Build history of the part. All positions in model axes, mm. A direction names the side the tool comes from. Round coordinates to 2 decimals unless told otherwise and drop trailing zeros. Write each loop counter-clockwise with the first axis right and the second up, starting at its lowest first coordinate (ties: lowest second). Pieces come first, ordered by that corner, then holes. Notation, with made-up numbers: M 0,52 L 5,52 A24 cw 5,66 Z; hole C 74.5,75.5 d5. An arc over 180 degrees is marked long. Write item = value, one per line. Start each with the question number.
Q1. Band-saw the part on D-D on x = 62. Write the cut outline in (y, z).
Q2. Pull direction Y, two halves, no side cores. Call faces 1 (the flat face through (48, 10, 110)), 2 (the cylindrical face through (76.48, 12.87, 133.07)), 3 (the flat face through (0, 86, 8)): released by +Y, released by -Y, zero draft, split by the parting line, or undercut.
Q3. Band-saw the part on C-C on y = 79. Write the cut outline in (x, z), plus the area to 3 significant figures.
Q4. Band-saw the part on A-A on x = 21. Write the cut outline in (y, z), plus the area to 3 significant figures.
Q5. Probe L1, parallel to Y at x = 3.2, z = 30; L2, parallel to Y at x = 1.2, z = 5. List the from-to ranges inside material, lowest first.
Q6. Band-saw the part on B-B on z = 73.5. Write the cut outline in (x, y), plus the area to 3 significant figures.
Q7. Drop flat-ended pins along their axis: P1, Ø2.5, axis at x = 76, z = 34, coming from the +Y side; P2, Ø0.9, axis at x = 76.5, z = 99.5, coming from the -Y side; P3, Ø2.5, axis at y = 145.5, z = 120.5, coming from the -X side; P4, Ø0.9, axis at y = 12, z = 106.5, coming from the -X side. Give the stop position or say it passes through.
Q8. Tool access for faces 4 (the flat face through (50, 5, 110)), 5 (the cylindrical face through (76.48, 17.32, 11.63)), 6 (the flat face through (48, 17, 12)): list every direction of +Z, -Z, +X, -X, +Y, -Y with a clear straight run to the whole face (end or side of a thin tool).
Autodesk Inventor part; units mm, degrees
ref_plane "YZ Plane" through (0, 0, 0) normal (1, 0, 0) x (0, 1, 0)
ref_plane "XZ Plane" through (0, 0, 0) normal (0, 1, 0) x (-1, 0, 0)
ref_plane "XY Plane" through (0, 0, 0) normal (0, 0, 1) x (1, 0, 0)
sketch "Sketch1" plane through (0, 0, 0) normal (0, 0, 1) x (1, 0, 0)
  line L0 (0, 0) -> (75, 0)
  line L1 (75, 0) -> (75, 150)
  line L2 (75, 150) -> (0, 150)
  line L3 (0, 150) -> (0, 0)
  dimension "d0" = 75
  dimension "d1" = 150
extrude "Extrusion1" add sketch "Sketch1" along normal blind 10
sketch "Sketch2" plane through (0, 0, 10) normal (0, 0, 1) x (1, 0, 0)
  line L0 (48, 85) -> (53, 85)
  line L1 (53, 85) -> (53, 19)
  line L2 (53, 19) -> (48, 19)
  line L3 (48, 19) -> (48, 14)
  line L4 (48, 14) -> (58, 14)
  line L5 (58, 14) -> (58, 90)
  line L6 (58, 90) -> (48, 90)
  line L7 (75, 150) -> (0, 150)
  line L8 (0, 150) -> (0, 0)
  line L9 (48, 85) -> (48, 90)
  dimension "d4" = 10
  dimension "d5" = 76
  dimension "d6" = 66
  dimension "d8" = 60
  dimension "d9" = 5
  dimension "d10" = 10
  dimension "d11" = 53
  dimension "d12" = 5
  dimension "d13" = 5
extrude "Extrusion2" add sketch "Sketch2" along normal blind 5
sketch "Sketch3" plane through (53, 19, 10) normal (-1, 0, 0) x (0, 0, 1)
  line L0 (5, 66) -> (5, 0)
  line L1 (5, 66) -> (3, 66)
  line L2 (3, 66) -> (3, 56)
  line L3 (3, 56) -> (5, 56)
  line L4 (5, 56) -> (5, 66)
  line L5 (5, 0) -> (5, -5)
  line L6 (5, 0) -> (3, 0)
  line L7 (3, 0) -> (3, 10)
  line L8 (3, 10) -> (5, 10)
  line L9 (5, 10) -> (5, 0)
  point P0 (-10, -19)
  point P1 (5, 10)
  point P2 (5, 56)
  dimension "d16" = 2
  dimension "d17" = 10
  dimension "d18" = 10
  dimension "d19" = 2
extrude "Extrusion3" add sketch "Sketch3" along normal blind 3
sketch "Sketch4" plane through (0, 0, 10) normal (0, 0, 1) x (1, 0, 0)
  line L0 (0, 150) -> (0, 0)
  line L1 (0, 10) -> (65, 10)
  line L2 (65, 10) -> (65, 140)
  line L3 (65, 140) -> (0, 140)
  line L4 (75, 150) -> (0, 150)
  line L5 (75, 0) -> (75, 150)
  line L6 (0, 0) -> (75, 0)
  point P0 (0, 140)
  dimension "d22" = 10
  dimension "d24" = 10
  dimension "d25" = 10
extrude "Extrusion4" add sketch "Sketch4" along normal blind 140 contours L4 L5 L6 L0 L1 L2 L3
sketch "Sketch5" plane through (0, 10, 10) normal (0, 1, 0) x (1, 0, 0)
  line L0 (0, 10) -> (0, -140)
  line L1 (0, -115) -> (50, -115)
  line L2 (50, -115) -> (50, -85)
  line L3 (50, -85) -> (0, -85)
  line L4 (0, -115) -> (0, -120)
  line L5 (0, -120) -> (55, -120)
  line L6 (55, -120) -> (55, -80)
  line L7 (55, -80) -> (0, -80)
  line L8 (0, -85) -> (0, -80)
  line L9 (0, -140) -> (75, -140)
  dimension "d28" = 50
  dimension "d29" = 30
  dimension "d30" = 5
  dimension "d31" = 55
  dimension "d32" = 40
  dimension "d37" = 20
extrude "Extrusion5" add sketch "Sketch5" along normal blind 10 contours L7 L6 L5 L0 L1 L2 L3
sketch "Sketch6" plane through (0, 10, 95) normal (0, 1, 0) x (1, 0, 0)
  line L0 (50, -30) -> (50, 0)
  line L1 (0, 0) -> (0, -30)
  line L2 (50, -30) -> (0, -30)
  line L3 (0, -30) -> (0, 0)
  line L4 (0, 0) -> (50, 0)
  line L5 (50, 0) -> (50, -30)
  point P0 (0, 95)
  point P1 (0, -30)
extrude "Extrusion6" cut sketch "Sketch6" against normal blind 10
sketch "Sketch7" plane through (50, 0, 125) normal (-1, 0, 0) x (0, 0, 1)
  line L0 (-30, 0) -> (-30, 20)
  line L1 (0, 20) -> (0, 0)
  line L2 (-30, 20) -> (0, 20)
  line L3 (0, 20) -> (0, 17)
  line L4 (0, 17) -> (-30, 17)
  line L5 (-30, 17) -> (-30, 20)
  line L6 (0, 10) -> (-30, 10)
  line L7 (-30, 10) -> (-30, 13)
  line L8 (-30, 13) -> (0, 13)
  line L9 (0, 13) -> (0, 10)
  point P0 (-125, 0)
  point P1 (0, 13)
  point P2 (-30, 13)
  point P3 (0, 20)
  dimension "d38" = 3
  dimension "d39" = 3
extrude "Extrusion7" add sketch "Sketch7" along normal blind 5 contours L0 L8 L1 L6 | L0 L2 L1 L4
sketch "Sketch8" plane through (0, 0, 0) normal (-1, 0, 0) x (0, 0, 1)
  circle A0 centre (5, 120) radius 2.5
  circle A1 centre (5, 30) radius 2.5
  circle A2 centre (60, 5) radius 2.5
  circle A3 centre (120, 145) radius 2.5
  circle A4 centre (30, 145) radius 2.5
  line L0 (0, 0) -> (95, 0)
  line L1 (0, 150) -> (0, 0)
  line L2 (0, 150) -> (150, 150)
  line L3 (10, 140) -> (150, 140)
  line L4 (150, 150) -> (150, 140)
  dimension "d42" = 5
  dimension "d43" = 5
  dimension "d44" = 5
  dimension "d45" = 5
  dimension "d46" = 5
  dimension "d47" = 5
  dimension "d48" = 60
  dimension "d49" = 5
  dimension "d50" = 30
  dimension "d51" = 5
  dimension "d52" = 30
  dimension "d53" = 30
  dimension "d54" = 5
  dimension "d55" = 5
  dimension "d56" = 30
extrude "Extrusion8" cut sketch "Sketch8" against normal blind 5
sketch "Sketch9" plane through (75, 0, 0) normal (1, 0, 0) x (0, 0, -1)
  line L0 (-92, 25.5) -> (-92, 55.5)
  line L1 (-92, 55.5) -> (-111, 55.5)
  line L2 (-111, 55.5) -> (-111, 85.5)
  line L3 (-111, 85.5) -> (-92, 85.5)
  line L4 (-92, 85.5) -> (-92, 72.5)
  line L5 (-92, 72.5) -> (-81.582, 62.082)
  line L6 (-81.582, 62.082) -> (-51.582, 62.082)
  line L7 (-51.582, 62.082) -> (-51.582, 92.082)
  line L8 (-51.582, 92.082) -> (-70.582, 92.082)
  line L9 (-70.582, 92.082) -> (-70.582, 111.082)
  line L10 (-70.582, 111.082) -> (-80, 120.5)
  line L11 (-80, 120.5) -> (-121, 120.5)
  line L12 (-135, 38.5) -> (-122, 25.5)
  line L13 (-122, 25.5) -> (-92, 25.5)
  line L14 (-41.582, 62.082) -> (-22.582, 62.082)
  line L15 (-22.582, 62.082) -> (-22.582, 92.082)
  line L16 (-22.582, 92.082) -> (-41.582, 92.082)
  line L17 (-41.582, 92.082) -> (-41.582, 62.082)
  line L18 (-150, 0) -> (-150, 150)
  line L19 (0, 150) -> (-150, 150)
  line L20 (-135, 38.5) -> (-135, 101.5)
  line L21 (-135, 101.5) -> (-121, 120.5)
  line L22 (-10, 10) -> (-150, 10)
  circle A0 centre (-140, 10) radius 7.5
  line L23 (-10, 140) -> (-150, 140)
  circle A1 centre (-140, 140) radius 7.5
  line L24 (-10, 10) -> (-90, 10)
  circle A2 centre (-10, 10) radius 7.5
  line L25 (-10, 140) -> (-10, 10)
  circle A3 centre (-10, 140) radius 7.5
  line L26 (0, 0) -> (0, 150)
  point P0 (-100.5, 120.5)
  point P1 (-51.582, 77.082)
  point P2 (-135, 70)
  dimension "d59" = 30
  dimension "d60" = 19
  dimension "d61" = 30
  dimension "d62" = 19
  dimension "d63" = 13
  dimension "d64" = 30
  dimension "d65" = 30
  dimension "d66" = 19
  dimension "d67" = 19
  dimension "d68" = 41
  dimension "d69" = 30
  dimension "d76" = 13
  dimension "d80" = 19
  dimension "d81" = 10
  dimension "d85" = 95
  dimension "d86" = 63
  dimension "d87" = 80
  dimension "d88" = 15
  dimension "d89" = 15
  dimension "d90" = 15
  dimension "d91" = 15
  dimension "d92" = 15
  dimension "d93" = 10
  dimension "d94" = 10
  dimension "d95" = 10
extrude "Extrusion9" add sketch "Sketch9" along normal blind 3 contours L13 L12 L20 L21 L11 L10 L9 L8 L7 L6 L5 L4 L3 L2 L1 L0 | L17 L16 L15 L14 | A0 L22 | L22 A0 | A1 L23 | L23 A1 | A3 L25 L23 | L23 L25 A3 | A2 L25 L22 | L22 L25 A2
properties part number "vraagblok2"
Conclusion:
q1.outline = M 0,0 L 150,0 L 150,150 L 140,150 L 140,10 L 10,10 L 10,150 L 0,150 Z
q2.face_1 = released by -Y
q2.face_2 = undercut
q2.face_3 = zero draft
q3.outline = M 0,0 L 75,0 L 75,22.58 L 78,22.58 L 78,41.58 L 75,41.58 L 75,51.58 L 78,51.58 L 78,92 L 75,92 L 75,111 L 78,111 L 78,135 L 75,135 L 75,150 L 65,150 L 65,10 L 58,10 L 58,15 L 50,15 L 50,13 L 53,13 L 53,10 L 0,10 Z
q3.area = 2,430 mm^2
q4.outline = M 0,0 L 150,0 L 150,150 L 140,150 L 140,10 L 10,10 L 10,90 L 20,90 L 20,95 L 0,95 Z; M 0,125 L 20,125 L 20,130 L 10,130 L 10,150 L 0,150 Z
q4.area = 4,100 mm^2
q5.L1 = 0 to 10, 140 to 142.5, 147.5 to 150
q5.L2 = 0 to 27.5, 32.5 to 117.5, 122.5 to 150
q6.outline = M 0,0 L 75,0 L 75,62.08 L 78,62.08 L 78,114 L 75,114 L 75,150 L 0,150 L 0,140 L 65,140 L 65,10 L 0,10 Z
q6.area = 2,960 mm^2
q7.P1 = 150
q7.P2 = 25.5
q7.P3 = 5
q7.P4 = 45
q8.face_4 = -X, -Y
q8.face_5 = +X
q8.face_6 = -X
